```python
from build123d import *

# Parameters (mm, degrees)
BOX_W        = 10
BOX_H        = 10
BOX_DEPTH    = 10
SKETCH_R     = 4
POCKET_DEPTH = 15
SKETCH001_R  = 1.94
PAD_DEPTH    = 10


with BuildPart() as part:
    # Box → Box (new body)
    with BuildSketch(Plane.XY):
        with Locations((5, 5)):
            Rectangle(BOX_W, BOX_H)
    extrude(amount=BOX_DEPTH)

    # Sketch (on Face6 of BaseFeature) → Pocket (cut)
    with BuildSketch(Plane.XY.offset(10)):
        with Locations((5, 5)):
            Circle(SKETCH_R)
    extrude(amount=-POCKET_DEPTH, mode=Mode.SUBTRACT)

    # Sketch001 (on Face4 of Pocket) → Pad (join)
    with BuildSketch(Plane(origin=(0, 10, 0), x_dir=(-1, 0, 0), z_dir=(0, 1, 0))):
        with Locations((-5, 5)):
            Circle(SKETCH001_R)
    extrude(amount=PAD_DEPTH)


solid = part.part
```
For this review, take the finished solid that the model builds, in its own axes (mm). A direction names the side the tool comes from. Give positions to 0.01 mm unless a question says otherwise; leave off trailing zeros. Loops run counter-clockwise (first coordinate to the right, second up) from the corner with the lowest first, then second, coordinate; pieces in that order, holes last. Notation, with made-up numbers: M 14.25,5 L 57.25,5 A28 ccw 57.25,23 Z; hole C -13.75,-22 d11. An arc over 180 degrees is marked long. One line per item, written item: value. Start each with the question number.
Q1. Draft analysis for pull direction Y (two halves, no side actions). For faces 1 (the face through (4.133, 1.095, 5.07)), 2 (the face through (5.253, 14.93, 6.923)), 3 (the face through (5, 0, 5)), 4 (the face through (5, 20, 5)), state which applies: released by +Y, released by -Y, zero draft, split by the parting line, or undercut.
Q2. Machinability: for faces 5 (the face through (0, 5, 5)), 6 (the face through (7.2, 10, 4.9)), which of the approach directions +Z, -Z, +X, -X, +Y, -Y give a long, thin tool a straight path to every point of the face, cutting with its end or side? Answer none if there is none.
Q3. Add section C-C (x = 5). Give the boundary of the cut face in (y, z).
Q4. Clearance check with flat-ended pins moving along their axes: pin 1 Ø2 at (x, z) = (2, 7.5) entering from +Y; pin 2 Ø4 at (x, y) = (6, 17.5) entering from +Z. State where each tip first meets the part, or that it passes through.
Q5. For L1, parallel to Y at x = 5, z = 3.25; L2, parallel to Y at x = 5, z = 2.5; L3, parallel to X at y = 2, z = 3.75, list the stretches that pass through material, from the lowest coordinate up.
Q6. Add section A-A (z = 5). Give the boundary of the cut face in (x, y), and give its area (3 significant figures).
Q7. Add section D-D (x = 6.5). Give the boundary of the cut face in (y, z), and give its area (3 significant figures).
Q8. Add section B-B (y = 5). Give the boundary of the cut face in (x, z).
Reply:
1. face 1: undercut
1. face 2: zero draft
1. face 3: released by -Y
1. face 4: released by +Y
2. face 5: +Z, -Z, -X, +Y, -Y
2. face 6: +Y
3. outline: M 0,0 L 1,0 L 1,10 L 0,10 Z; M 9,0 L 10,0 L 10,3.06 L 20,3.06 L 20,6.94 L 10,6.94 L 10,10 L 9,10 Z
4. pin 1: y = 10
4. pin 2: z = 6.94
5. L1: 0 to 1, 9 to 20
5. L2: 0 to 1, 9 to 10
5. L3: 0 to 2.35, 7.65 to 10
6. outline: M 0,0 L 10,0 L 10,10 L 6.94,10 L 6.94,20 L 3.06,20 L 3.06,10 L 0,10 Z; hole C 5,5 d8
6. area: 88.5 mm²
7. outline: M 0,0 L 1.29,0 L 1.29,10 L 0,10 Z; M 8.71,0 L 10,0 L 10,3.77 L 20,3.77 L 20,6.23 L 10,6.23 L 10,10 L 8.71,10 Z
7. area: 50.4 mm²
8. outline: M 0,0 L 1,0 L 1,10 L 0,10 Z; M 9,0 L 10,0 L 10,10 L 9,10 Z
